```python
from build123d import *

# Parameters (mm, degrees)
SKETCH1_W           = 260
SKETCH1_H           = 260
BOSS_EXTRUDE1_DEPTH = 30
SKETCH2_R           = 10
BOSS_EXTRUDE2_DEPTH = 10
BOSS_EXTRUDE3_DEPTH = 50
FILLET1_R           = 10


with BuildPart() as part:
    # Sketch1 → Boss-Extrude1 (new body)
    with BuildSketch(Plane.XY):
        with Locations((70.296296296, -67.888888889)):
            Rectangle(SKETCH1_W, SKETCH1_H)
    extrude(amount=BOSS_EXTRUDE1_DEPTH)

    # Sketch2 → Boss-Extrude2 (add)
    with BuildSketch(Plane(origin=(200.296296296, 0, 0), x_dir=(0, 0, -1), z_dir=(1, 0, 0))):
        with Locations(Location((-20, -187.888888889, 0), (0, 0, 180))):
            Circle(SKETCH2_R)
    extrude(amount=BOSS_EXTRUDE2_DEPTH)

    # Sketch3 → Boss-Extrude3 (add)
    with BuildSketch(Plane(origin=(0, 62.111111111, 0), x_dir=(1, 0, 0), z_dir=(0, 1, 0))):
        with BuildLine():
            Line((-59.703703704, 0), (200.296296296, 0))
            ThreePointArc((200.296296296, 0), (70.296296296, 29.629883308), (-59.703703704, 0))
        make_face()
    extrude(amount=-BOSS_EXTRUDE3_DEPTH)

    # Fillet1
    fillet1_edges = [part.edges().sort_by_distance(p)[0] for p in [
        (70.296296296, -197.888888889, 30),
        (70.296296296, -197.888888889, 0),
    ]]
    fillet(fillet1_edges, radius=FILLET1_R)

    # Sketch5 → Cut-Revolve1 (revolve, cut)
    with BuildSketch(Plane(origin=(0, 0, -30), x_dir=(-1, 0, 0), z_dir=(0, 0, -1))):
        with BuildLine():
            Line((-111.130147267, 62.111111111), (-29.462445326, 62.111111111))
            ThreePointArc((-29.462445326, 62.111111111), (-70.296296296, 83.256360811), (-111.130147267, 62.111111111))
        make_face()
    revolve(axis=Axis((111.130147267, 62.111111111, -30), (-1, 0, 0)), mode=Mode.SUBTRACT)

    # Sketch6 → Cut-Revolve2 (revolve, cut)
    with BuildSketch(Plane(origin=(0, 0, -30), x_dir=(-1, 0, 0), z_dir=(0, 0, -1))):
        with BuildLine():
            Line((-168.914289208, 12.111111111), (28.321696616, 12.111111111))
            ThreePointArc((28.321696616, 12.111111111), (-70.296296296, -10.693397865), (-168.914289208, 12.111111111))
        make_face()
    revolve(axis=Axis((168.914289208, 12.111111111, -30), (-1, 0, 0)), mode=Mode.SUBTRACT)


solid = part.part
```
For this review, take the finished solid that the model builds, in its own axes (mm). A direction names the side the tool comes from. Coordinates: 2 decimals unless noted, no trailing zeros. Write each loop counter-clockwise with the first axis right and the second up, starting at its lowest first coordinate (ties: lowest second). Pieces come first, ordered by that corner, then holes. Notation, with made-up numbers: (58.25, 4) - (102.25, 4) arc R20 cw to (102.25, 29) - close; hole circle Ø2 at (84.25, -16). An arc over 180 degrees is marked (long way). Answer in a Markdown table with one row per item. Add a question column.
Q1. For probe 1 along Y at (x, z) = (15, -2.5); probe 2 along Z at (x, y) = (147, -71.5); probe 3 along X at (y, z) = (-33.5, 13.5), list the stretches that pass through material, from the lowest coordinate up.
Q2. Tool access review of faces 1 (the cylindrical face through (72.179, 37.461, -29.624)), 2 (the cylindrical face through (205.226, -178.127, 17.832)), 3 (the flat face through (68, -86, 0)): name each direction out of +Z, -Z, +X, -X, +Y, -Y from which nothing blocks a thin tool from reaching the whole face with its end or side.
Q3. We need section A-A, the plane x = -39.5. State the section outline as (y, z) points, and give its area (3 significant figures).
Q4. We need section C-C, the plane y = -46. State the section outline as (x, z) points, and give its area (3 significant figures).
Q5. We need section B-B, the plane z = 15. State the section outline as (x, y) points, and give its area (3 significant figures).
Q6. For P1, Ø12, axis at x = -30, z = -23, coming from the -Y side; P2, Ø6, axis at x = 42, z = -7, coming from the -Y side; P3, Ø24, axis at y = -18, z = 10, coming from the +X side; P4, Ø5, axis at x = 92.5, z = 3.5, coming from the -Y side, all flat-tipped, find the tip position at first contact; note any pin that passes through.
Answer list:
| question | item | result |
|---|---|---|
| 1 | probe 1 | y = 12.11 to 62.11 |
| 1 | probe 2 | z = 0 to 30 |
| 1 | probe 3 | x = -59.7 to 200.3 |
| 2 | face 1 | -Z, +Y, -Y |
| 2 | face 2 | +X |
| 2 | face 3 | -Z, +X, -X, -Y |
| 3 | outline | (-197.89, 10) arc R10 ccw to (-187.89, 0) - (12.11, 0) - (12.11, -8.82) - (62.11, -8.82) - (62.11, 30) - (-187.89, 30) arc R10 ccw to (-197.89, 20) - close |
| 3 | area | 8,200 mm2 |
| 4 | outline | (-59.7, 0) - (200.3, 0) - (200.3, 30) - (-59.7, 30) - close |
| 4 | area | 7,800 mm2 |
| 5 | outline | (-59.7, -197.89) - (200.3, -197.89) - (200.3, -196.55) - (210.3, -196.55) - (210.3, -179.23) - (200.3, -179.23) - (200.3, 62.11) - (-59.7, 62.11) - close |
| 5 | area | 67,800 mm2 |
| 6 | P1 | passes through |
| 6 | P2 | stops at y = 12.11 |
| 6 | P3 | stops at x = 200.3 |
| 6 | P4 | stops at y = -197.05 |
